Check sheet for the drawn part. Datum: minimum x, y, z corner. Units: mm. Round coordinates to 2 decimals unless told otherwise and drop trailing zeros. Order: outer loops, then holes, each group sorted by start corner. A loop starts at its lowest first (then second) coordinate and runs counter-clockwise, first axis right, second up. Notation, with made-up numbers: (34, 35) -> (87, 35) arc R23 cw to (87, 57) -> close; hole circle Ø3 at (-38, 71.25). An arc over 180 degrees is marked (long way). Use CSV: the item, a comma, the result in double quotes.
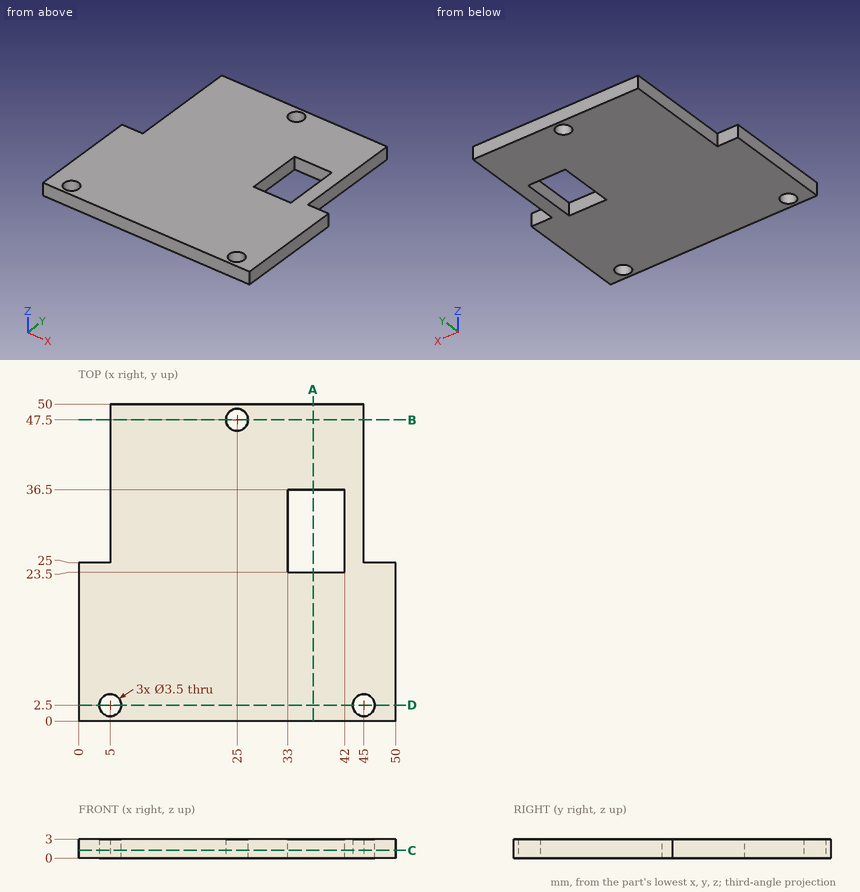
Q1. Scan lines: L1, parallel to X at y = 2.5, z = 1.6; L2, parallel to X at y = 47.5, z = 1.05; L3, parallel to X at y = 28.5, z = 0.75. Record each from-to range of solid material in increasing order.
Result sheet:
L1,"x = 0 to 3.25, 6.75 to 43.25, 46.75 to 50"
L2,"x = 5 to 23.25, 26.75 to 45"
L3,"x = 5 to 33, 42 to 45"
Q2. Sectioned sample at B-B, the plane y = 47.5. Enter the section's corners in (x, z), then the cut area to 4 significant figures.
Result sheet:
outline,"(5, 0) -> (23.25, 0) -> (23.25, 3) -> (5, 3) -> close; (26.75, 0) -> (45, 0) -> (45, 3) -> (26.75, 3) -> close"
area,"109.5 mm^2"
Q3. Sectioned sample at D-D, the plane y = 2.5. Enter the section's corners in (x, z).
Result sheet:
outline,"(0, 0) -> (3.25, 0) -> (3.25, 3) -> (0, 3) -> close; (6.75, 0) -> (43.25, 0) -> (43.25, 3) -> (6.75, 3) -> close; (46.75, 0) -> (50, 0) -> (50, 3) -> (46.75, 3) -> close"
Q4. Sectioned sample at C-C, the plane z = 1.2. Enter the section's corners in (x, y), then the cut area to 3 significant figures.
Result sheet:
outline,"(0, 0) -> (50, 0) -> (50, 25) -> (45, 25) -> (45, 50) -> (5, 50) -> (5, 25) -> (0, 25) -> close; hole circle Ø3.5 at (5, 2.5); hole circle Ø3.5 at (25, 47.5); hole (33, 23.5) -> (42, 23.5) -> (42, 36.5) -> (33, 36.5) -> close; hole circle Ø3.5 at (45, 2.5)"
area,"2,100 mm^2"
Q5. Sectioned sample at A-A, the plane x = 37. Enter the section's corners in (y, z), then the cut area to 3 significant figures.
Result sheet:
outline,"(0, 0) -> (23.5, 0) -> (23.5, 3) -> (0, 3) -> close; (36.5, 0) -> (50, 0) -> (50, 3) -> (36.5, 3) -> close"
area,"111 mm^2"
Q6. Go/stop test with flat-tipped pins: pin 1 (1.5 mm diameter, centred on x = 1.5, z = 1.5, fed in from +Y); pin 2 (0.9 mm diameter, centred on y = 39.5, z = 2, fed in from +X); pin 3 (2 mm diameter, centred on x = 5, y = 2.5, fed in from -Z). Record where each tip stops, or that it passes through.
Result sheet:
pin 1,"stops at y = 25"
pin 2,"stops at x = 45"
pin 3,"passes through"
